The model under review builds one solid part; all positions refer to its coordinate system, in mm. A direction names the side the tool comes from. Coordinates: 2 decimals unless noted, no trailing zeros. Write each loop counter-clockwise with the first axis right and the second up, starting at its lowest first coordinate (ties: lowest second). Pieces come first, ordered by that corner, then holes. Notation, with made-up numbers: (69.5, -3) - (104.5, -3) arc R24 cw to (104.5, 34) - close; hole circle Ø1 at (45, 83). An arc over 180 degrees is marked (long way). Put each result on its own line as item: value. Start each with the question number.
Item 1: Mouldability with a two-part tool opening along X and no side actions: class faces 1 (the face through (-3.375, 2, 4)), 2 (the face through (-10, 0, 3)), 3 (the face through (0, 0, 8)) as pulls with the +X half, pulls with the -X half, needs draft (parallel to the pull), parting line crosses it, or undercut.
Item 2: To check wall thickness, follow L1, parallel to Y at x = -1, z = 5.5 (3 decimals); L2, parallel to X at y = 0, z = 6; L3, parallel to X at y = 1, z = 1 (3 decimals). State the ranges of each line that lie inside material, in increasing order. Write a range as [from, to].
Item 3: For pin 1 (3 mm diameter, centred on x = -6.5, y = 0, fed in from +Z); pin 2 (1 mm diameter, centred on y = 2.5, z = 1.5, fed in from -X); pin 3 (0.8 mm diameter, centred on y = 2.5, z = 4.5, fed in from +X); pin 4 (2 mm diameter, centred on y = -2, z = 4, fed in from +X), all flat-tipped, find the tip position at first contact; note any pin that passes through.
Item 4: Consider section A-A on y = 0. Give the boundary of the cut face in (x, z).
Item 5: Machinability: for faces 4 (the face through (6, -2, 4)), 5 (the face through (3.375, -2, 4)), 6 (the face through (0, -4, 3)), which of the approach directions +Z, -Z, +X, -X, +Y, -Y give a long, thin tool a straight path to every point of the face, cutting with its end or side? Answer none if there is none.
```python
from build123d import *

# Parameters (mm, degrees)
F0_W        = 6.75
F0_H        = 2.75
F0_R        = 1.75
F1_DEPTH    = 8
F2_R        = 3
F2_R_2      = 1.75
F3_DEPTH    = 4
F4_T1_DEPTH = 12
F4_T4_ANGLE = 180
F4_T6_ANGLE = 180


# Not quite as in the source:
# - a fillet or chamfer that OpenCascade refuses, or shapes differently, is made with other operations: its cross-section is extruded or revolved along the edge and cut away or added


with BuildPart() as f1:
    # F0 (on Top) → F1 (new body)
    with BuildSketch(Plane.XY):
        with BuildLine():
            ThreePointArc((6, -4), (10, 0), (6, 4))
            Line((6, 4), (-6, 4))
            ThreePointArc((-6, 4), (-10, 0), (-6, -4))
            Line((-6, -4), (6, -4))
        make_face()
        with Locations((0, -2)):
            Rectangle(F0_W, F0_H, mode=Mode.SUBTRACT)
        with Locations((-6.5, 0)):
            Circle(F0_R, mode=Mode.SUBTRACT)
        with Locations((6.5, 0)):
            Circle(F0_R, mode=Mode.SUBTRACT)
        with Locations((0, 2)):
            Rectangle(F0_W, F0_H, mode=Mode.SUBTRACT)
    extrude(amount=F1_DEPTH)

    # F2 (on face) → F3 (cut)
    with BuildSketch(Plane.XY.offset(8)):
        with Locations((-6.5, 0)):
            Circle(F2_R)
        with Locations((-6.5, 0)):
            Circle(F2_R_2, mode=Mode.SUBTRACT)
        with Locations((6.5, 0)):
            Circle(F2_R)
        with Locations((6.5, 0)):
            Circle(F2_R_2, mode=Mode.SUBTRACT)
    extrude(amount=-F3_DEPTH, mode=Mode.SUBTRACT)

    # F4: fillet of radius 1 on 1 edges, made by hand

    # F4_s2 → F4_t1 (cut)
    with BuildSketch(Plane.YZ.offset(-6)):
        with BuildLine():
            ThreePointArc((-4, 7), (-3.7071067812, 7.7071067812), (-3, 8))
            Line((-3, 8), (-4, 8))
            Line((-4, 8), (-4, 7))
        make_face()
        with BuildLine():
            ThreePointArc((3, 8), (3.7071067812, 7.7071067812), (4, 7))
            Line((4, 7), (4, 8))
            Line((4, 8), (3, 8))
        make_face()
    extrude(amount=F4_T1_DEPTH, mode=Mode.SUBTRACT)

    # F4_s3 → F4_t4 (revolve, cut)
    with BuildSketch(Plane.YZ.offset(6)):
        with BuildLine():
            ThreePointArc((-4, 7), (-3.7071067812, 7.7071067812), (-3, 8))
            Line((-3, 8), (-4, 8))
            Line((-4, 8), (-4, 7))
        make_face()
    revolve(axis=Axis((6, 0, 8), (0, 0, 1)), revolution_arc=F4_T4_ANGLE, mode=Mode.SUBTRACT)

    # F4_s5 → F4_t6 (revolve, cut)
    with BuildSketch(Plane.YZ.offset(-6)):
        with BuildLine():
            ThreePointArc((4, 7), (3.7071067812, 7.7071067812), (3, 8))
            Line((3, 8), (4, 8))
            Line((4, 8), (4, 7))
        make_face()
    revolve(axis=Axis((-6, 0, 8), (0, 0, 1)), revolution_arc=F4_T6_ANGLE, mode=Mode.SUBTRACT)


solid = f1.part
```
Report:
1. face 1: undercut
1. face 2: pulls with the -X half
1. face 3: needs draft
2. L1: [-4, -3.375], [-0.625, 0.625], [3.375, 4]
2. L2: [-10, -9.5], [-3.5, 3.5], [9.5, 10]
2. L3: [-9.873, -7.936], [-5.064, -3.375], [3.375, 5.064], [7.936, 9.873]
3. pin 1: through
3. pin 2: x = -9.46
3. pin 3: x = 9.4
3. pin 4: x = 9.87
4. outline: (-10, 0) - (-8.25, 0) - (-8.25, 4) - (-9.5, 4) - (-9.5, 7.87) arc R1 ccw to (-10, 7) - close; (-4.75, 0) - (4.75, 0) - (4.75, 4) - (3.5, 4) - (3.5, 8) - (-3.5, 8) - (-3.5, 4) - (-4.75, 4) - close; (8.25, 0) - (10, 0) - (10, 7) arc R1 ccw to (9.5, 7.87) - (9.5, 4) - (8.25, 4) - close
5. face 4: +Z
5. face 5: +Z, -Z
5. face 6: +Z, -Z, +X, -X, -Y
